The listing builds one solid part. Answer for the finished solid, in the listing's coordinates (mm). Face numbers are marked on the shaded views. A direction names the side the tool comes from. Give positions to 0.01 mm unless a question says otherwise; leave off trailing zeros. Order: outer loops, then holes, each group sorted by start corner. A loop starts at its lowest first (then second) coordinate and runs counter-clockwise, first axis right, second up.
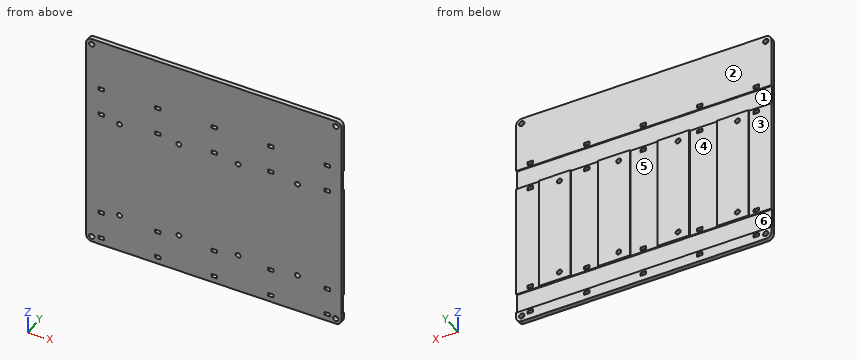
```python
from build123d import *

# Parameters (mm, degrees)
BODY_SKETCH_W                          = 230
BODY_SKETCH_H                          = 200
BODY_DEPTH                             = 4
MOUNTING_HOLES_OUTLINE_R               = 2.4
MOUNTING_HOLES_DEPTH                   = 4
SKETCH4_W                              = 230
SKETCH4_H                              = 18
CABLE_CUTOUTS_DEPTH                    = 1
SKETCH6_W                              = 28.5
SKETCH6_H                              = 104
DRIVER_EXTRUSION_DEPTH                 = 1
DRIVER_MOUNTING_HOLES_OUTLINE_R        = 2.25
DRIVER_MOUNTING_HOLES_DEPTH            = 5
DRIVER_PATTERN_COUNT                   = 4
DRIVER_PATTERN_PITCH                   = 53.5
SKETCH9_W                              = 5
SKETCH9_H                              = 3
CABLE_FIXIATOR_CUTOUT_DEPTH            = 153.449991801
CABLE_FIXIATOR_PATTERN_COUNT           = 5
CABLE_FIXIATOR_PATTERN_PITCH           = 51
CABLE_FIXIATOR_PATTERN_COPY_1_SKETCH_W = 5
CABLE_FIXIATOR_PATTERN_COPY_1_SKETCH_H = 3
CABLE_FIXIATOR_PATTERN_COPY_1_DEPTH    = 153.449991801
CABLE_FIXIATOR_PATTERN_COPY_2_SKETCH_W = 5
CABLE_FIXIATOR_PATTERN_COPY_2_SKETCH_H = 3
CABLE_FIXIATOR_PATTERN_COPY_2_DEPTH    = 153.449991801
CABLE_FIXIATOR_PATTERN_COPY_3_SKETCH_W = 5
CABLE_FIXIATOR_PATTERN_COPY_3_SKETCH_H = 3
CABLE_FIXIATOR_PATTERN_COPY_3_DEPTH    = 153.449991801
CABLE_FIXIATOR_PATTERN_COPY_4_SKETCH_W = 5
CABLE_FIXIATOR_PATTERN_COPY_4_SKETCH_H = 3
CABLE_FIXIATOR_PATTERN_COPY_4_DEPTH    = 153.449991801
EDGE_FILLETS_R                         = 5


# Read off the part's stored shape, not the designer's step: mounting_holes, driver_mounting_holes
with BuildPart() as part:
    # body_sketch → body (new body)
    with BuildSketch(Plane(origin=(0, 0, 0), x_dir=(1, 0, 0), z_dir=(0, 1, 0))):
        Rectangle(BODY_SKETCH_W, BODY_SKETCH_H)
    extrude(amount=BODY_DEPTH)

    # mounting_holes outline → mounting_holes (cut)
    with BuildSketch(Plane(origin=(0, 0, 0), x_dir=(1, 0, 0), z_dir=(0, 1, 0))):
        with Locations((110, -95)):
            Circle(MOUNTING_HOLES_OUTLINE_R)
        with Locations((-110, 95)):
            Circle(MOUNTING_HOLES_OUTLINE_R)
        with Locations((-110, -95)):
            Circle(MOUNTING_HOLES_OUTLINE_R)
        with Locations((110, 95)):
            Circle(MOUNTING_HOLES_OUTLINE_R)
    extrude(amount=MOUNTING_HOLES_DEPTH, mode=Mode.SUBTRACT)

    # Sketch4 → cable_cutouts (cut)
    with BuildSketch(Plane(origin=(0, 4, 0), x_dir=(1, 0, 0), z_dir=(0, 1, 0))):
        with Locations((0, 81)):
            Rectangle(SKETCH4_W, SKETCH4_H)
        with Locations((0, -41)):
            Rectangle(SKETCH4_W, SKETCH4_H)
    extrude(amount=-CABLE_CUTOUTS_DEPTH, mode=Mode.SUBTRACT)

    # Sketch6 → driver_extrusion (add)
    with BuildSketch(Plane(origin=(0, 4, 0), x_dir=(1, 0, 0), z_dir=(0, 1, 0))):
        with Locations((-80.75, 20)):
            Rectangle(SKETCH6_W, SKETCH6_H)
    driver_extrusion = extrude(amount=DRIVER_EXTRUSION_DEPTH)

    # driver_mounting_holes outline → driver_mounting_holes (cut)
    with BuildSketch(Plane(origin=(0, 0, 0), x_dir=(1, 0, 0), z_dir=(0, 1, 0))):
        with Locations((-85, -25)):
            Circle(DRIVER_MOUNTING_HOLES_OUTLINE_R)
        with Locations((-85, 65)):
            Circle(DRIVER_MOUNTING_HOLES_OUTLINE_R)
    driver_mounting_holes = extrude(amount=DRIVER_MOUNTING_HOLES_DEPTH, mode=Mode.SUBTRACT)

    # driver_pattern: driver_extrusion, driver_mounting_holes ×4
    with Locations(*[(i * DRIVER_PATTERN_PITCH, 0, 0) for i in range(1, DRIVER_PATTERN_COUNT)]):
        add(driver_extrusion)
        add(driver_mounting_holes, mode=Mode.SUBTRACT)

    # Sketch9 → cable_fixiator_cutout (cut, through all)
    with BuildSketch(Plane(origin=(0, 4, 0), x_dir=(1, 0, 0), z_dir=(0, 1, 0))):
        with Locations((-101.5, 93.5)):
            Rectangle(SKETCH9_W, SKETCH9_H)
        with Locations((-101.5, 68.5)):
            Rectangle(SKETCH9_W, SKETCH9_H)
    cable_fixiator_cutout = extrude(amount=-CABLE_FIXIATOR_CUTOUT_DEPTH, mode=Mode.SUBTRACT)

    # cable_fixiator_mirror: cable_fixiator_cutout across plane
    add(cable_fixiator_cutout.mirror(Plane.XY.offset(-20)), mode=Mode.SUBTRACT)

    # cable_fixiator_pattern: cable_fixiator_cutout ×5
    with Locations(*[(i * CABLE_FIXIATOR_PATTERN_PITCH, 0, 0) for i in range(1, CABLE_FIXIATOR_PATTERN_COUNT)]):
        add(cable_fixiator_cutout, mode=Mode.SUBTRACT)

    # cable_fixiator_pattern copy 1 sketch → cable_fixiator_pattern copy 1 (cut, through all)
    with BuildSketch(Plane(origin=(51, 4, -40), x_dir=(1, 0, 0), z_dir=(0, 1, 0))):
        with Locations((-101.5, -93.5)):
            Rectangle(CABLE_FIXIATOR_PATTERN_COPY_1_SKETCH_W, CABLE_FIXIATOR_PATTERN_COPY_1_SKETCH_H)
        with Locations((-101.5, -68.5)):
            Rectangle(CABLE_FIXIATOR_PATTERN_COPY_1_SKETCH_W, CABLE_FIXIATOR_PATTERN_COPY_1_SKETCH_H)
    extrude(amount=-CABLE_FIXIATOR_PATTERN_COPY_1_DEPTH, mode=Mode.SUBTRACT)

    # cable_fixiator_pattern copy 2 sketch → cable_fixiator_pattern copy 2 (cut, through all)
    with BuildSketch(Plane(origin=(102, 4, -40), x_dir=(1, 0, 0), z_dir=(0, 1, 0))):
        with Locations((-101.5, -93.5)):
            Rectangle(CABLE_FIXIATOR_PATTERN_COPY_2_SKETCH_W, CABLE_FIXIATOR_PATTERN_COPY_2_SKETCH_H)
        with Locations((-101.5, -68.5)):
            Rectangle(CABLE_FIXIATOR_PATTERN_COPY_2_SKETCH_W, CABLE_FIXIATOR_PATTERN_COPY_2_SKETCH_H)
    extrude(amount=-CABLE_FIXIATOR_PATTERN_COPY_2_DEPTH, mode=Mode.SUBTRACT)

    # cable_fixiator_pattern copy 3 sketch → cable_fixiator_pattern copy 3 (cut, through all)
    with BuildSketch(Plane(origin=(153, 4, -40), x_dir=(1, 0, 0), z_dir=(0, 1, 0))):
        with Locations((-101.5, -93.5)):
            Rectangle(CABLE_FIXIATOR_PATTERN_COPY_3_SKETCH_W, CABLE_FIXIATOR_PATTERN_COPY_3_SKETCH_H)
        with Locations((-101.5, -68.5)):
            Rectangle(CABLE_FIXIATOR_PATTERN_COPY_3_SKETCH_W, CABLE_FIXIATOR_PATTERN_COPY_3_SKETCH_H)
    extrude(amount=-CABLE_FIXIATOR_PATTERN_COPY_3_DEPTH, mode=Mode.SUBTRACT)

    # cable_fixiator_pattern copy 4 sketch → cable_fixiator_pattern copy 4 (cut, through all)
    with BuildSketch(Plane(origin=(204, 4, -40), x_dir=(1, 0, 0), z_dir=(0, 1, 0))):
        with Locations((-101.5, -93.5)):
            Rectangle(CABLE_FIXIATOR_PATTERN_COPY_4_SKETCH_W, CABLE_FIXIATOR_PATTERN_COPY_4_SKETCH_H)
        with Locations((-101.5, -68.5)):
            Rectangle(CABLE_FIXIATOR_PATTERN_COPY_4_SKETCH_W, CABLE_FIXIATOR_PATTERN_COPY_4_SKETCH_H)
    extrude(amount=-CABLE_FIXIATOR_PATTERN_COPY_4_DEPTH, mode=Mode.SUBTRACT)

    # edge_fillets
    edge_fillets_edges = [part.edges().sort_by_distance(p)[0] for p in [
        (115, 2, 100),
        (-115, 2, 100),
        (-115, 2, -100),
        (115, 2, -100),
    ]]
    fillet(edge_fillets_edges, radius=EDGE_FILLETS_R)


solid = part.part
```
1) For a pull along X with two mould halves and no side action, classify the marked faces 5 and 6 as +X half, -X half, draft (parallel to the pull), parting line (faces both ways), or undercut.
Geometry says:
face 5: undercut
face 6: draft
2) Given P1, Ø0.5, axis at y = 4.5, z = -30, coming from the -X side; P2, Ø15, axis at x = -15, z = 66, coming from the +Y side; P3, Ø4.5, axis at x = -110, z = 95, coming from the -Y side, each flat-ended and moving along its own axis, determine where each tip first touches the part or whether it passes through.
Geometry says:
P1: stops at x = -95
P2: stops at y = 4
P3: passes through
3) Straight lines are drawn through the part: probe 1 along Z at (x, y) = (75.5, 2); probe 2 along Z at (x, y) = (110, 1.3); probe 3 along X at (y, z) = (4.6, -13). For each, find the intervals that lie inside material, in ascending order.
Geometry says:
probe 1: z = -100 to -67.25, -62.75 to 22.75, 27.25 to 100
probe 2: z = -100 to -97.4, -92.6 to 92.6, 97.4 to 100
probe 3: x = -95 to -66.5, -41.5 to -13, 12 to 40.5, 65.5 to 94
4) Find section A-A (x = 7). Write down the section's boundary in (y, z).
Geometry says:
outline: (0, -100) - (4, -100) - (4, -90) - (3, -90) - (3, -72) - (4, -72) - (4, 32) - (3, 32) - (3, 50) - (4, 50) - (4, 100) - (0, 100) - close
5) Find section C-C (x = 90). Write down the section's boundary in (y, z).
Geometry says:
outline: (0, -100) - (4, -100) - (4, -90) - (3, -90) - (3, -72) - (5, -72) - (5, 32) - (3, 32) - (3, 50) - (4, 50) - (4, 100) - (0, 100) - close
6) A tool of negligible diameter and unlimited length cuts with its end or side. For the marked faces 1, 2, 3 and 4, from which of +Z, -Z, +X, -X, +Y, -Y can it reach the whole face along a straight path? Write none if from no direction.
Geometry says:
face 1: +X, -X, +Y
face 2: +Z, +X, -X, +Y
face 3: +Z, -Z, -X, +Y
face 4: +Z, -Z, +Y
7) Find section B-B (z = -19). Write down the section's boundary in (x, y), then the cut area to 3 significant figures.
Geometry says:
outline: (-115, 0) - (115, 0) - (115, 4) - (94, 4) - (94, 5) - (65.5, 5) - (65.5, 4) - (40.5, 4) - (40.5, 5) - (12, 5) - (12, 4) - (-13, 4) - (-13, 5) - (-41.5, 5) - (-41.5, 4) - (-66.5, 4) - (-66.5, 5) - (-95, 5) - (-95, 4) - (-115, 4) - close
area: 1,030 mm2
